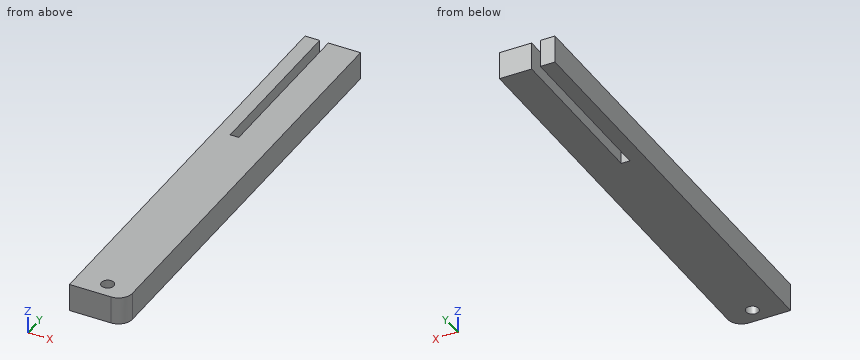
from build123d import *

# Parameters (mm, degrees)
SKETCH1_W           = 10.16
SKETCH1_H           = 80.800676527
BOSS_EXTRUDE1_DEPTH = 5.08
FILLET1_R           = 2.54
SKETCH2_R           = 1.143
SKETCH2_W           = 1.579389271
SKETCH2_H           = 30.704752465
CUT_EXTRUDE1_DEPTH  = 5.08


with BuildPart() as part:
    # Sketch1 → Boss-Extrude1 (new body)
    with BuildSketch(Plane.XY):
        with Locations((-3.236775432, 33.601000469)):
            Rectangle(SKETCH1_W, SKETCH1_H)
    extrude(amount=BOSS_EXTRUDE1_DEPTH)

    # Fillet1
    fillet1_edges = [part.edges().sort_by_distance(p)[0] for p in [
        (1.843224568, -6.799337795, 2.54),
    ]]
    fillet(fillet1_edges, radius=FILLET1_R)

    # Sketch2 → Cut-Extrude1 (cut)
    with BuildSketch(Plane.XY.offset(5.08)):
        with Locations((-2.915125323, -3.81)):
            Circle(SKETCH2_R)
        with Locations((-4.845930623, 58.6489625)):
            Rectangle(SKETCH2_W, SKETCH2_H)
    extrude(amount=-CUT_EXTRUDE1_DEPTH, mode=Mode.SUBTRACT)


solid = part.part
Check sheet for the modelled part. Datum: model origin and axes. Units: mm. Round coordinates to 2 decimals unless told otherwise and drop trailing zeros. Order: outer loops, then holes, each group sorted by start corner. A loop starts at its lowest first (then second) coordinate and runs counter-clockwise, first axis right, second up.
Q1. Cross-section at B-B, the plane x = -4.75. Enter the section's corners in (y, z), plus the area to 3 significant figures.
Filled sheet:
outline: (-6.8, 0) - (43.3, 0) - (43.3, 5.08) - (-6.8, 5.08) - close
area: 254 mm2
Q2. Scan lines: L1, parallel to Y at x = -3, z = 3.9; L2, parallel to X at y = 52, z = 3.95; L3, parallel to Y at x = -2.25, z = 1.5. Record each from-to range of solid material in increasing order.
Filled sheet:
L1: y = -6.8 to -4.95, -2.67 to 74
L2: x = -8.32 to -5.64, -4.06 to 1.84
L3: y = -6.8 to -4.74, -2.88 to 74
Q3. Cross-section at A-A, the plane z = 3.7. Enter the section's corners in (x, y).
Filled sheet:
outline: (-8.32, -6.8) - (-0.7, -6.8) arc R2.54 ccw to (1.84, -4.26) - (1.84, 74) - (-4.06, 74) - (-4.06, 43.3) - (-5.64, 43.3) - (-5.64, 74) - (-8.32, 74) - close; hole circle Ø2.29 at (-2.92, -3.81)
